Part model, mm, in its own coordinate system. Give positions to 0.01 mm unless a question says otherwise; leave off trailing zeros. Answer in a Markdown table with one row per item. Add a question column.
1. Probe line 1 along X through (y, z) = (7.2, 30); line 2 along X through (y, z) = (1.45, 510). List the from-to ranges inside material, lowest first.
2. Band-saw the part on A-A on y = 2. State how many separate pieces and enclosed holes the cut face has, plus the area to 3 significant figures.
3. Drop a flat-ended pin along its axis: pin 1 Ø3 at (x, z) = (6.5, 670.5) entering from +Y. Give the stop position or say it passes through.
```python
from build123d import *

# Parameters (mm, degrees)
SKETCH1_W                      = 15
SKETCH1_H                      = 10
BOSS_EXTRUDE1_DEPTH            = 700
CBORE_FOR_M3_SHCS1_D           = 3.5
CBORE_FOR_M3_SHCS1_CBORE_D     = 6
CBORE_FOR_M3_SHCS1_CBORE_DEPTH = 4.5
LPATTERN1_COUNT                = 17
LPATTERN1_PITCH                = 40


with BuildPart() as part:
    # Sketch1 → Boss-Extrude1 (new body)
    with BuildSketch(Plane.XY):
        with Locations((7.5, 5)):
            Rectangle(SKETCH1_W, SKETCH1_H)
    extrude(amount=BOSS_EXTRUDE1_DEPTH)

    # CBORE for M3 SHCS1 (through all)
    with Locations(Plane(origin=(0, 10, 0), x_dir=(1, 0, 0), z_dir=(0, 1, 0))):
        with Locations((7.5, -670)):
            cbore_for_m3_shcs1 = CounterBoreHole(CBORE_FOR_M3_SHCS1_D / 2, CBORE_FOR_M3_SHCS1_CBORE_D / 2, CBORE_FOR_M3_SHCS1_CBORE_DEPTH)

    # LPattern1: CBORE for M3 SHCS1 ×17
    with Locations(*[(0, 0, -i * LPATTERN1_PITCH) for i in range(1, LPATTERN1_COUNT)]):
        add(cbore_for_m3_shcs1, mode=Mode.SUBTRACT)


solid = part.part
```
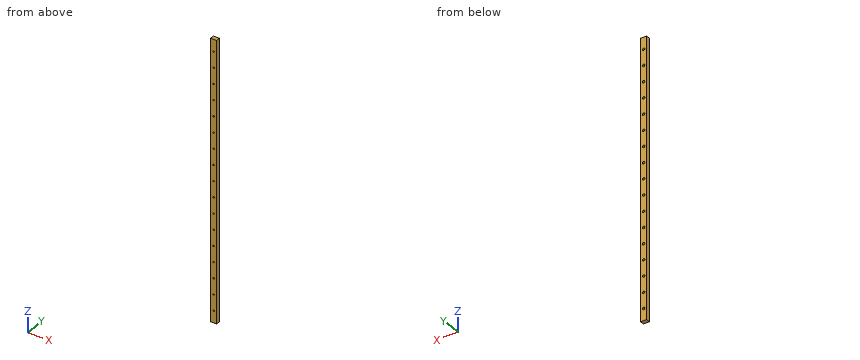
Values:
| question | item | result |
|---|---|---|
| 1 | line 1 | x = 0 to 4.5, 10.5 to 15 |
| 1 | line 2 | x = 0 to 5.75, 9.25 to 15 |
| 2 | separate pieces | 1 |
| 2 | enclosed holes | 17 |
| 2 | area | 10,300 mm² |
| 3 | pin 1 | stops at y = 5.5 |
